from build123d import *

# Parameters (mm, degrees)
SKETCH1_R           = 2
BOSS_EXTRUDE1_DEPTH = 100
LPATTERN1_COUNT     = 2
LPATTERN1_PITCH     = 20


with BuildPart() as part:
    # Sketch1 → Boss-Extrude1 (new body)
    with BuildSketch(Plane.XY):
        Polygon((-10, 3.075), (-8.15, 3.075), (-8.15, 5.95), (-6.91873629, 5.95), (-3.75, 2.78126371), (-3.75, 0), (-3.75, -2.78126371), (-6.91873629, -5.95), (-8.15, -5.95), (-8.15, -3.075), (-10, -3.075), (-10, -10), (-3.075, -10), (-3.075, -8.15), (-5.95, -8.15), (-5.95, -6.91873629), (-2.78126371, -3.75), (0, -3.75), (2.78126371, -3.75), (5.95, -6.91873629), (5.95, -8.15), (3.075, -8.15), (3.075, -10), (10, -10), (10, -3.075), (8.15, -3.075), (8.15, -5.95), (6.91873629, -5.95), (3.75, -2.78126371), (3.75, 0), (3.75, 2.78126371), (6.91873629, 5.95), (8.15, 5.95), (8.15, 3.075), (10, 3.075), (10, 10), (3.075, 10), (3.075, 8.15), (5.95, 8.15), (5.95, 6.91873629), (2.78126371, 3.75), (0, 3.75), (-2.78126371, 3.75), (-5.95, 6.91873629), (-5.95, 8.15), (-3.075, 8.15), (-3.075, 10), (-10, 10), align=None)
        Circle(SKETCH1_R, mode=Mode.SUBTRACT)
    boss_extrude1 = extrude(amount=BOSS_EXTRUDE1_DEPTH)

    # LPattern1: Boss-Extrude1 ×2
    with Locations(*[(0, i * LPATTERN1_PITCH, 0) for i in range(1, LPATTERN1_COUNT)]):
        add(boss_extrude1)


solid = part.part
Could you check a few things on this model? Use its own coordinates, in mm. A direction names the side the tool comes from. Give positions to 0.01 mm unless a question says otherwise; leave off trailing zeros. Order: outer loops, then holes, each group sorted by start corner. A loop starts at its lowest first (then second) coordinate and runs counter-clockwise, first axis right, second up.
Item 1: If we section it at B-B, the plane x = 0: Write out the boundary of the cut face in (y, z).
Item 2: If we section it at A-A, the plane y = 0: Write out the boundary of the cut face in (x, z).
Item 3: If we mould it in two halves opening along X, with no side actions, what happens to faces 1 (the face through (10, -7, 49)), 2 (the face through (-9, 16.925, 49)), 3 (the face through (5.31, 24.34, 49.3))? For each: pulls with the +X half, pulls with the -X half, needs draft (parallel to the pull), parting line crosses it, or undercut.
Item 4: I need wall thicknesses on line 1 (Y direction, x = 0, z = 25); line 2 (Y direction, x = -8.25, z = 55) (3 decimals); line 3 (X direction, y = 15, z = 26.5). Which ranges of each line are inside material? Lowest first, please.
Item 5: I'm going to push flat-ended pins straight in: pin 1 (1.7 mm diameter, centred on x = 0, z = 40, fed in from -Y); pin 2 (4.5 mm diameter, centred on y = 19.5, z = 71.5, fed in from -X); pin 3 (3 mm diameter, centred on y = 0.5, z = 50.5, fed in from +X); pin 4 (3 mm diameter, centred on x = -1, y = 7, fed in from -Z). Where does each tip first touch, or does it pass through?
Item 6: If we section it at C-C, the plane z = 58: Count the separate pieces of the cut face and the enclosed holes in it, plus the area to 3 significant figures.
Item 7: For faces 4 (the face through (0, 23.75, 49)), 5 (the face through (-9, 23.075, 49)), 6 (the face through (4, 10, 0)), 7 (the face through (9, 16.925, 49)), 8 (the face through (3.075, 10, 49)), which set-ups out of +Z, -Z, +X, -X, +Y, -Y let a thin tool reach every point of the face, with its end or its side?
Values:
1. outline: (-3.75, 0) - (-2, 0) - (-2, 100) - (-3.75, 100) - close; (2, 0) - (3.75, 0) - (3.75, 100) - (2, 100) - close; (16.25, 0) - (18, 0) - (18, 100) - (16.25, 100) - close; (22, 0) - (23.75, 0) - (23.75, 100) - (22, 100) - close
2. outline: (-3.75, 0) - (-2, 0) - (-2, 100) - (-3.75, 100) - close; (2, 0) - (3.75, 0) - (3.75, 100) - (2, 100) - close
3. face 1: pulls with the +X half
3. face 2: needs draft
3. face 3: undercut
4. line 1: y = -3.75 to -2, 2 to 3.75, 16.25 to 18, 22 to 23.75
4. line 2: y = -10 to -3.075, 3.075 to 16.925, 23.075 to 30
4. line 3: x = -10 to -8.15, -5.97 to -4.03, 4.03 to 5.97, 8.15 to 10
5. pin 1: stops at y = -3.75
5. pin 2: stops at x = -3.75
5. pin 3: stops at x = 3.75
5. pin 4: passes through
6. separate pieces: 1
6. enclosed holes: 3
6. area: 345 mm2
7. face 4: +Z, -Z, +Y
7. face 5: +Z, -Z, -X
7. face 6: -Z, +X, -X, +Y, -Y
7. face 7: +Z, -Z, +X
7. face 8: +Z, -Z
